Could you check a few things on this model? Use its own coordinates, in mm. Face numbers are marked on the shaded views. A direction names the side the tool comes from. Give positions to 0.01 mm unless a question says otherwise; leave off trailing zeros. Loops run counter-clockwise (first coordinate to the right, second up) from the corner with the lowest first, then second, coordinate; pieces in that order, holes last. Notation, with made-up numbers: M -20.5,65.25 L 15.5,65.25 A33 cw 15.5,94.25 Z; hole C 46,16.5 d9. An arc over 180 degrees is marked long. Answer in a Markdown table with one row per item. Add a question column.
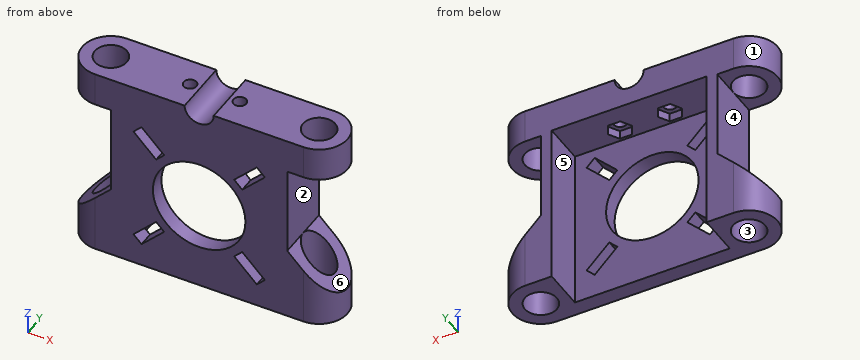
```python
from build123d import *

# Parameters (mm, degrees)
SCHIZZO1_R        = 4.5
BASE_DEPTH        = 27.5
HOLES_START       = -16
HOLES_OUTLINE_R   = 13
HOLES_DEPTH       = 16
SCHIZZO5_W        = 43.5
SCHIZZO5_H        = 46
FLANGE_DEPTH      = 11.7
SCREW_HOLES_REACH = 68.907
SCHIZZO6_R        = 1.8
NUT_START         = -2.4
SCHIZZO7_R        = 1.8
NUT_HOLES_DEPTH   = 2.4


# Read off the part's stored shape, not the designer's step: Holes
with BuildPart() as part:
    # Schizzo1 → Base (new, symmetric)
    with BuildSketch(Plane.XY):
        with BuildLine():
            Line((-29.25, -8), (29.25, -8))
            ThreePointArc((29.25, -8), (37.25, 0), (29.25, 8))
            Line((29.25, 8), (-29.25, 8))
            ThreePointArc((-29.25, 8), (-37.25, 0), (-29.25, -8))
        make_face()
        with Locations((-29.25, 0)):
            Circle(SCHIZZO1_R, mode=Mode.SUBTRACT)
        with Locations(Location((29.25, 0, 0), (0, 0, 180))):
            Circle(SCHIZZO1_R, mode=Mode.SUBTRACT)
    extrude(amount=BASE_DEPTH, both=True)

    # Holes outline → Holes (cut)
    with BuildSketch(Plane(origin=(0, 8, 0), x_dir=(1, 0, 0), z_dir=(0, 1, 0)).offset(HOLES_START)):
        Polygon((9.828784258, 14.591525958), (12.091525958, 12.328784258), (18.455486989, 18.692745289), (16.192745289, 20.955486989), align=None)
        Polygon((24.75, -18), (37.25, -18), (37.25, 19.5), (24.75, 7), align=None)
        Polygon((-37.25, 19.5), (-37.25, -18), (-24.75, -18), (-24.75, 7), align=None)
        with BuildLine():
            Line((-4.09, -27.5), (4.09, -27.5))
            ThreePointArc((4.09, -27.5), (0, -23.41), (-4.09, -27.5))
        make_face()
        Polygon((-12.091525958, 12.328784258), (-9.828784258, 14.591525958), (-16.192745289, 20.955486989), (-18.455486989, 18.692745289), align=None)
        Polygon((12.091525958, -7.328784258), (9.828784258, -9.591525958), (16.192745289, -15.955486989), (18.455486989, -13.692745289), align=None)
        Polygon((-9.828784258, -9.591525958), (-12.091525958, -7.328784258), (-18.455486989, -13.692745289), (-16.192745289, -15.955486989), align=None)
        with Locations((0, 2.5)):
            Circle(HOLES_OUTLINE_R)
    extrude(amount=HOLES_DEPTH, mode=Mode.SUBTRACT)

    # Schizzo5 → Flange (cut)
    with BuildSketch(Plane(origin=(0, 8, 0), x_dir=(1, 0, 0), z_dir=(0, 1, 0))):
        with Locations((0, 4.5)):
            Rectangle(SCHIZZO5_W, SCHIZZO5_H)
    extrude(amount=-FLANGE_DEPTH, mode=Mode.SUBTRACT)

    # Schizzo6 → Screw holes (cut, up to next)
    with BuildSketch(Plane.XY.offset(27.5), mode=Mode.PRIVATE) as screw_holes_sk1:
        with Locations((7, 0)):
            Circle(SCHIZZO6_R)
    screw_holes_tool1 = extrude(screw_holes_sk1.sketch, amount=-SCREW_HOLES_REACH, mode=Mode.PRIVATE) & part.part
    # Schizzo6 → Screw holes (cut, up to next)
    with BuildSketch(Plane.XY.offset(27.5), mode=Mode.PRIVATE) as screw_holes_sk2:
        with Locations((-7, 0)):
            Circle(SCHIZZO6_R)
    screw_holes_tool2 = extrude(screw_holes_sk2.sketch, amount=-SCREW_HOLES_REACH, mode=Mode.PRIVATE) & part.part
    add(screw_holes_tool1.solids().sort_by_distance((7, 0, 27.5))[0], mode=Mode.SUBTRACT)
    add(screw_holes_tool2.solids().sort_by_distance((-7, 0, 27.5))[0], mode=Mode.SUBTRACT)

    # Schizzo7 → Nut holes (cut)
    # profile 1 of 2: a face of its own
    with BuildSketch(Plane(origin=(0, 0, 18.5), x_dir=(-1, 0, 0), z_dir=(0, 0, -1)).offset(NUT_START)):
        Polygon((-3.6, 0), (-5.3, 2.944486373), (-8.7, 2.944486373), (-10.4, 0), (-8.7, -2.944486373), (-5.3, -2.944486373), align=None)
    # profile 2 of 2: a face of its own
    with BuildSketch(Plane(origin=(0, 0, 18.5), x_dir=(-1, 0, 0), z_dir=(0, 0, -1)).offset(NUT_START)):
        Polygon((10.4, 0), (8.7, 2.944486373), (5.3, 2.944486373), (3.6, 0), (5.3, -2.944486373), (8.7, -2.944486373), align=None)
        with Locations((7, 0)):
            Circle(SCHIZZO7_R, mode=Mode.SUBTRACT)
    extrude(amount=NUT_HOLES_DEPTH, mode=Mode.SUBTRACT)


solid = part.part
```
Item 1: I need wall thicknesses on L1, parallel to Y at x = -29.25, z = 25; L2, parallel to X at y = -2.5, z = 8.5; L3, parallel to X at y = -6.2, z = -2.5. Which ranges of each line are inside material? Lowest first, please.
Item 2: Suppose I cut it at B-B (z = -2.5). List the corners of the cut face in (x, y) for me.
Item 3: Suppose I cut it at A-A (x = -15). List the corners of the cut face in (y, z) for me, then the cut area to 3 significant figures.
Item 4: Suppose I cut it at D-D (x = -27). List the corners of the cut face in (y, z) for me, then the cut area to 3 significant figures.
Item 5: For the marked faces 4, 5 and 6, which set-ups out of +Z, -Z, +X, -X, +Y, -Y let a thin tool reach every point of the face, with its end or its side?
Item 6: Suppose I cut it at C-C (x = 0). List the corners of the cut face in (y, z) for me.
Item 7: For P1, Ø2, axis at x = -18, y = -2, coming from the -Z side; P2, Ø3, axis at y = -6.5, z = -21, coming from the +X side (3 decimals); P3, Ø2, axis at x = 7, y = 0, coming from the +Z side; P4, Ø8, axis at x = -16.5, z = 4, coming from the +Y side, each with a flat end and sliding along its axis, tell me the tip position at first contact or that it passes through.
Item 8: If we mould it in two halves opening along X, with no side actions, what happens to the marked faces 1, 2 and 3? For each: +X half, -X half, draft (parallel to the pull), parting line (faces both ways), or undercut.
Values found:
| question | item | result |
|---|---|---|
| 1 | L1 | -8 to -4.5, 4.5 to 8 |
| 1 | L2 | -24.75 to -21.75, 21.75 to 24.75 |
| 1 | L3 | -24.75 to -13, 13 to 24.75 |
| 2 | outline | M -24.75,-8 L -13,-8 L -13,-3.7 L -21.75,-3.7 L -21.75,8 L -24.75,8 Z; M 13,-8 L 24.75,-8 L 24.75,8 L 21.75,8 L 21.75,-3.7 L 13,-3.7 Z |
| 3 | outline | M -8,-27.5 L -3.7,-27.5 L -3.7,-19.76 L -8,-19.76 Z; M -8,-15.24 L -3.7,-15.24 L -3.7,10.24 L -8,10.24 Z; M -8,14.76 L -3.7,14.76 L -3.7,18.5 L 8,18.5 L 8,27.5 L -8,27.5 Z |
| 3 | area | 303 mm² |
| 4 | outline | M -8,-27.5 L -3.9,-27.5 L -3.9,-9.25 L -8,-9.25 Z; M -8,18 L -3.9,18 L -3.9,27.5 L -8,27.5 Z; M 3.9,-27.5 L 8,-27.5 L 8,-9.25 L 3.9,-9.25 Z; M 3.9,18 L 8,18 L 8,27.5 L 3.9,27.5 Z |
| 4 | area | 228 mm² |
| 5 | face 4 | -X, +Y, -Y |
| 5 | face 5 | -Z, +Y |
| 5 | face 6 | +X, +Y, -Y |
| 6 | outline | M -8,-27.5 L -3.7,-27.5 L -3.7,-15.5 L -8,-15.5 Z; M -8,10.5 L -3.7,10.5 L -3.7,18.5 L 8,18.5 L 8,23.41 L -8,23.41 Z |
| 7 | P1 | z = 18.5 |
| 7 | P2 | x = 35.495 |
| 7 | P3 | through |
| 7 | P4 | y = -3.7 |
| 8 | face 1 | -X half |
| 8 | face 2 | +X half |
| 8 | face 3 | undercut |
